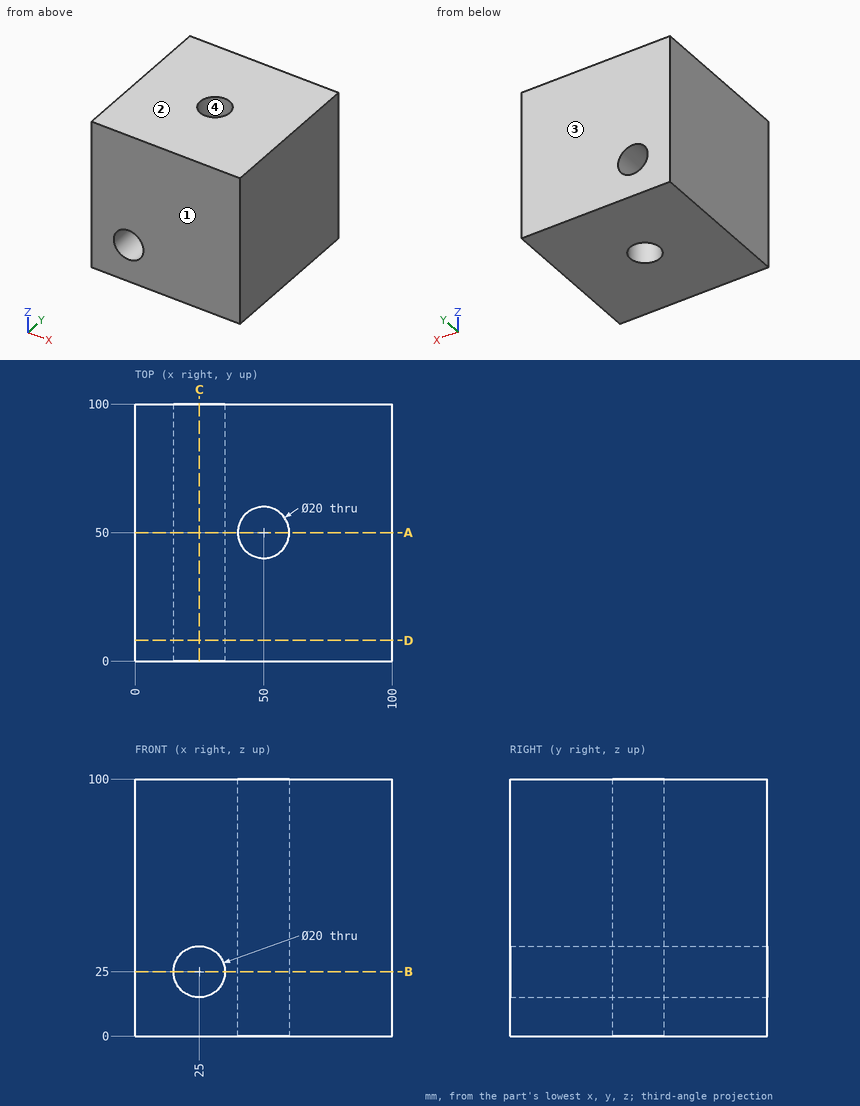
For this review, use the dimensioned drawing (mm, ordinates from the lowest corner) and the shaded views. Round coordinates to 2 decimals unless told otherwise and drop trailing zeros. Order: outer loops, then holes, each group sorted by start corner. A loop starts at its lowest first (then second) coordinate and runs counter-clockwise, first axis right, second up. Notation, with made-up numbers: M -39,-31.5 L -35,-31.5 A16 ccw -35,-2.5 Z; hole C 86,-35.5 d8. An arc over 180 degrees is marked long. Use a Markdown table: item, result. Add a question column.
Item 1: Mouldability with a two-part tool opening along Y and no side actions: class the marked faces 1, 2, 3 and 4 as released by +Y, released by -Y, zero draft, split by the parting line, or undercut.
Item 2: Add section D-D, the plane y = 8. Give the boundary of the cut face in (x, z), then the cut area to 3 significant figures.
Item 3: Add section B-B, the plane z = 25. Give the boundary of the cut face in (x, y).
Item 4: Add section A-A, the plane y = 50. Give the boundary of the cut face in (x, z).
Item 5: Add section C-C, the plane x = 25. Give the boundary of the cut face in (y, z).
Item 6: To check wall thickness, follow line 1 along X through (y, z) = (69.5, 25); line 2 along X through (y, z) = (18, 22). State the ranges of each line that lie inside material, in increasing order.
Geometry results:
| question | item | result |
|---|---|---|
| 1 | face 1 | released by -Y |
| 1 | face 2 | zero draft |
| 1 | face 3 | released by +Y |
| 1 | face 4 | undercut |
| 2 | outline | M 0,0 L 100,0 L 100,100 L 0,100 Z; hole C 25,25 d20 |
| 2 | area | 9,690 mm² |
| 3 | outline | M 0,0 L 15,0 L 15,100 L 0,100 Z; M 35,0 L 100,0 L 100,100 L 35,100 Z; hole C 50,50 d20 |
| 4 | outline | M 0,0 L 40,0 L 40,100 L 0,100 Z; M 60,0 L 100,0 L 100,100 L 60,100 Z; hole C 25,25 d20 |
| 5 | outline | M 0,0 L 100,0 L 100,15 L 0,15 Z; M 0,35 L 100,35 L 100,100 L 0,100 Z |
| 6 | line 1 | x = 0 to 15, 35 to 100 |
| 6 | line 2 | x = 0 to 15.46, 34.54 to 100 |
